Geometry check sheet. Reference: the model listing, model coordinates, mm. Give positions to 0.01 mm unless a question says otherwise; leave off trailing zeros. Write each loop counter-clockwise with the first axis right and the second up, starting at its lowest first coordinate (ties: lowest second). Pieces come first, ordered by that corner, then holes.
(1) Cross-section at C-C (x = -9.5). Record the boundary of the cut face in (y, z).
(2) Cross-section at D-D (x = -33.5). Record the boundary of the cut face in (y, z).
(3) Cross-section at A-A (y = 0). Record the boundary of the cut face in (x, z).
(4) Thickness scan on line 1 along Y through (x, z) = (-33.5, 0.7); line 2 along X through (y, z) = (2, 1.8); line 3 along X through (y, z) = (-3, 1). Record the ranges inside material, lowest first.
(5) Cross-section at B-B (z = 1.2). Record the boundary of the cut face in (x, y), and give its area (3 significant figures).
(6) Depth check by flat-ended pin: P1, Ø6.5, axis at x = -33.25, y = 0, coming from the +Z side; P2, Ø6.5, axis at x = 16.25, y = 0, coming from the +Z side. Enter the tip coordinate at first touch or a pass-through.
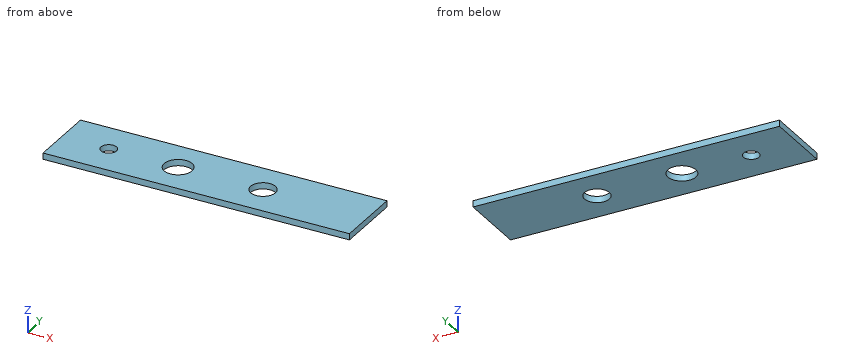
```python
from build123d import *

# Parameters (mm, degrees)
F1_W     = 98.332082
F1_H     = 22
F1_R     = 4.5
F1_R_2   = 4
F2_DEPTH = 2
F3_R     = 2.5
F4_DEPTH = 25


with BuildPart() as f2:
    # F1 (on face) → F2 (new body)
    with BuildSketch(Plane.XY):
        with Locations((0.833959, 0)):
            Rectangle(F1_W, F1_H)
        with Locations((-11.0046, 0)):
            Circle(F1_R, mode=Mode.SUBTRACT)
        with Locations((16.2454, 0)):
            Circle(F1_R_2, mode=Mode.SUBTRACT)
    extrude(amount=F2_DEPTH)

    # F3 (on face) → F4 (cut)
    with BuildSketch(Plane.XY.offset(2)):
        with Locations((-33.2546, 0)):
            Circle(F3_R)
    extrude(amount=-F4_DEPTH, mode=Mode.SUBTRACT)


solid = f2.part
```
Reply:
1. outline: (-11, 0) - (-4.24, 0) - (-4.24, 2) - (-11, 2) - close; (4.24, 0) - (11, 0) - (11, 2) - (4.24, 2) - close
2. outline: (-11, 0) - (-2.49, 0) - (-2.49, 2) - (-11, 2) - close; (2.49, 0) - (11, 0) - (11, 2) - (2.49, 2) - close
3. outline: (-48.33, 0) - (-35.75, 0) - (-35.75, 2) - (-48.33, 2) - close; (-30.75, 0) - (-15.5, 0) - (-15.5, 2) - (-30.75, 2) - close; (-6.5, 0) - (12.25, 0) - (12.25, 2) - (-6.5, 2) - close; (20.25, 0) - (50, 0) - (50, 2) - (20.25, 2) - close
4. line 1: y = -11 to -2.49, 2.49 to 11
4. line 2: x = -48.33 to -34.75, -31.75 to -15.04, -6.97 to 12.78, 19.71 to 50
4. line 3: x = -48.33 to -14.36, -7.65 to 13.6, 18.89 to 50
5. outline: (-48.33, -11) - (50, -11) - (50, 11) - (-48.33, 11) - close; hole circle Ø5 at (-33.25, 0); hole circle Ø9 at (-11, 0); hole circle Ø8 at (16.25, 0)
5. area: 2,030 mm2
6. P1: stops at z = 2
6. P2: passes through
